Could you check a few things on this model? Use its own coordinates, in mm. A direction names the side the tool comes from. Give positions to 0.01 mm unless a question says otherwise; leave off trailing zeros. Order: outer loops, then holes, each group sorted by start corner. A loop starts at its lowest first (then second) coordinate and runs counter-clockwise, first axis right, second up. Notation, with made-up numbers: (58, -19.5) -> (89, -19.5) arc R24 cw to (89, 7.5) -> close; hole circle Ø8 at (44, -9). An arc over 180 degrees is marked (long way). One line per item, written item: value.
```python
from build123d import *

# Parameters (mm, degrees)
SKETCH2_R           = 2.5
SKETCH2_R_2         = 2
BOSS_EXTRUDE2_DEPTH = 3


with BuildPart() as part:
    # Sketch2 → Boss-Extrude2 (new body)
    with BuildSketch(Plane(origin=(0, 0, 0), x_dir=(1, 0, 0), z_dir=(0, 1, 0))):
        with BuildLine():
            Line((10.594452967, -18.350130817), (45, -8))
            ThreePointArc((45, -8), (50.947530499, 0), (45, 8))
            Line((45, 8), (10.594452967, 18.350130817))
            Line((10.594452967, 18.350130817), (-15.57179677, 42.97114317))
            ThreePointArc((-15.57179677, 42.97114317), (-25.473765249, 44.121855672), (-29.42820323, 34.97114317))
            Line((-29.42820323, 34.97114317), (-21.188905934, 0))
            Line((-21.188905934, 0), (-29.42820323, -34.97114317))
            ThreePointArc((-29.42820323, -34.97114317), (-25.473765249, -44.121855672), (-15.57179677, -42.97114317))
            Line((-15.57179677, -42.97114317), (10.594452967, -18.350130817))
        make_face()
        with Locations(Location((0, 0, 0), (0, 0, 270))):
            Circle(SKETCH2_R, mode=Mode.SUBTRACT)
        with Locations(Location((-22.50172491, 38.974130802, 0), (0, 0, 270))):
            Circle(SKETCH2_R_2, mode=Mode.SUBTRACT)
        with Locations(Location((45.00344982, 0, 0), (0, 0, 270))):
            Circle(SKETCH2_R_2, mode=Mode.SUBTRACT)
        with Locations(Location((-22.50172491, -38.974130802, 0), (0, 0, 270))):
            Circle(SKETCH2_R_2, mode=Mode.SUBTRACT)
    extrude(amount=BOSS_EXTRUDE2_DEPTH)


solid = part.part
```
1) For faces 4 (the flat face through (-25.25, 1.48, 17.24)), 5 (the cylindrical face through (50.946, 1.479, 0.15)), which set-ups out of +Z, -Z, +X, -X, +Y, -Y let a thin tool reach every point of the face, with its end or its side?
Answer below:
face 4: -X, +Y, -Y
face 5: +X, +Y, -Y
2) Suppose I cut it at D-D, the plane x = 31.5. Write out the boundary of the cut face in (y, z).
Answer below:
outline: (0, -12.06) -> (3, -12.06) -> (3, 12.06) -> (0, 12.06) -> close
3) For P1, Ø1, axis at x = 38, y = 2.5, coming from the -Z side; P2, Ø1, axis at x = 0.5, y = 1, coming from the +Z side, each with a flat end and sliding along its axis, tell me the tip position at first contact or that it passes through.
Answer below:
P1: stops at z = -10.26
P2: stops at z = 28.32
4) Suppose I cut it at B-B, the plane x = 0. Write out the boundary of the cut face in (y, z).
Answer below:
outline: (0, -28.32) -> (3, -28.32) -> (3, -2.5) -> (0, -2.5) -> close; (0, 2.5) -> (3, 2.5) -> (3, 28.32) -> (0, 28.32) -> close
5) Suppose I cut it at A-A, the plane z = -39. Write out the boundary of the cut face in (x, y).
Answer below:
outline: (-29.38, 0) -> (-24.5, 0) -> (-24.5, 3) -> (-29.38, 3) -> close; (-20.5, 0) -> (-11.35, 0) -> (-11.35, 3) -> (-20.5, 3) -> close
6) If I drill on line 1 along Z through (x, y) = (46, 0.7); line 2 along Z through (x, y) = (32.5, 2.05); line 3 along Z through (x, y) = (26.5, 1.95), over which ranges is the centre line in solid material (lowest first)?
Answer below:
line 1: z = -7.63 to -1.73, 1.73 to 7.63
line 2: z = -11.76 to 11.76
line 3: z = -13.57 to 13.57
7) We'd pull the mould along Z, two halves only. Please class faces 1 (the flat face through (-2.67, 1.48, 30.83)), 2 (the flat face through (-8, 0, -1)), 3 (the flat face through (-25.366, 1.479, -17.73)): +Z half, -Z half, draft (parallel to the pull), parting line (faces both ways), or undercut.
Answer below:
face 1: +Z half
face 2: draft
face 3: undercut
8) Suppose I cut it at C-C, the plane y = 1.5. Write out the boundary of the cut face in (x, z).
Answer below:
outline: (-29.43, -34.97) arc R8.35 ccw to (-15.57, -42.97) -> (10.59, -18.35) -> (45, -8) arc R8.35 ccw to (45, 8) -> (10.59, 18.35) -> (-15.57, 42.97) arc R8.35 ccw to (-29.43, 34.97) -> (-21.19, 0) -> close; hole circle Ø4 at (-22.5, -38.97); hole circle Ø4 at (-22.5, 38.97); hole circle Ø5 at (0, 0); hole circle Ø4 at (45, 0)
